Verification items for this drawing (mm, ordinates from the low corner). A direction names the side the tool comes from. Round coordinates to 2 decimals unless told otherwise and drop trailing zeros. Order: outer loops, then holes, each group sorted by start corner. A loop starts at its lowest first (then second) coordinate and runs counter-clockwise, first axis right, second up. Notation, with made-up numbers: M 31.5,-32 L 46.5,-32 A21 cw 46.5,-3 Z; hole C 48.5,62.5 d3. An arc over 180 degrees is marked long. Return JSON: item names as keys, results as strings. Group by question number.
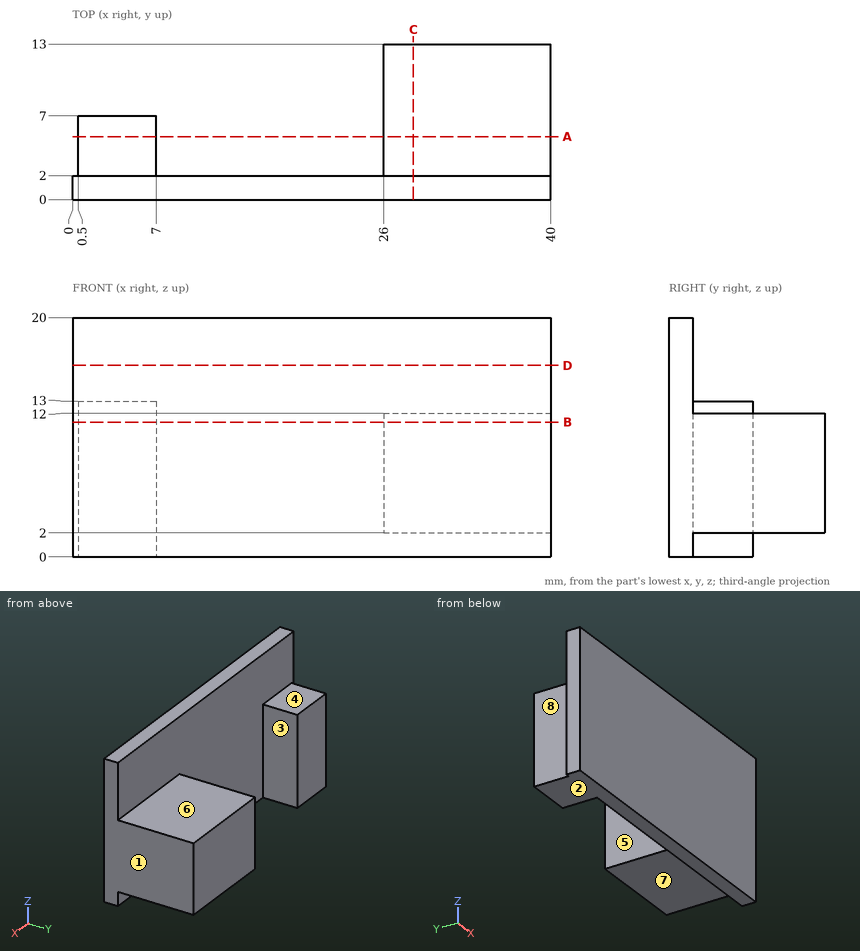
1. Draft check along X on the marked faces 1, 2 and 3. Enter one of: +X half, -X half, draft (parallel to the pull), parting line (faces both ways), or undercut.
2. Cross-section at D-D (z = 16). Enter the section's corners in (x, y), plus the area to 3 significant figures.
3. Thickness scan on line 1 along X through (y, z) = (5.5, 6.5); line 2 along Y through (x, z) = (11, 5); line 3 along Z through (x, y) = (37.5, 8.5). Record the ranges inside material, lowest first. Write a range as from..to.
4. Go/stop test with flat-tipped pins: pin 1 (5.5 mm diameter, centred on x = 30, y = 9, fed in from -Z); pin 2 (5.5 mm diameter, centred on x = 33.5, y = 9.5, fed in from +Z); pin 3 (1.5 mm diameter, centred on y = 4.5, z = 4, fed in from -X). Record where each tip stops, or that it passes through.
5. Cross-section at A-A (y = 5.25). Enter the section's corners in (x, z), plus the area to 4 significant figures.
6. Cross-section at B-B (z = 11.25). Enter the section's corners in (x, y).
7. Cross-section at C-C (x = 28.5). Enter the section's corners in (y, z).
8. Access from +Z, -Z, +X, -X, +Y, -Y to the whole of each face (thin tool, end or side, straight path). Record for the marked faces 4, 5, 6, 7 and 8.
Computed:
{
 "1": {"face 1": "+X half", "face 2": "draft", "face 3": "undercut"},
 "2": {"outline": "M 0,0 L 40,0 L 40,2 L 0,2 Z", "area": "80.0 mm²"},
 "3": {"line 1": "x = 0.5..7, 26..40", "line 2": "y = 0..2", "line 3": "z = 2..12"},
 "4": {"pin 1": "stops at z = 2", "pin 2": "stops at z = 12", "pin 3": "stops at x = 0.5"},
 "5": {"outline": "M 0.5,0 L 7,0 L 7,13 L 0.5,13 Z; M 26,2 L 40,2 L 40,12 L 26,12 Z", "area": "224.5 mm²"},
 "6": {"outline": "M 0,0 L 40,0 L 40,13 L 26,13 L 26,2 L 7,2 L 7,7 L 0.5,7 L 0.5,2 L 0,2 Z"},
 "7": {"outline": "M 0,0 L 2,0 L 2,2 L 13,2 L 13,12 L 2,12 L 2,20 L 0,20 Z"},
 "8": {"face 4": "+Z, +X, -X, +Y", "face 5": "+Z, -Z, +Y", "face 6": "+Z, +X, +Y", "face 7": "-Z, +X, +Y", "face 8": "+Z, -Z, -X, +Y"}
}
